Verification items for the finished model (mm, model axes). Face numbers are marked on the shaded views. A direction names the side the tool comes from. Round coordinates to 2 decimals unless told otherwise and drop trailing zeros. Loops run counter-clockwise (first coordinate to the right, second up) from the corner with the lowest first, then second, coordinate; pieces in that order, holes last.
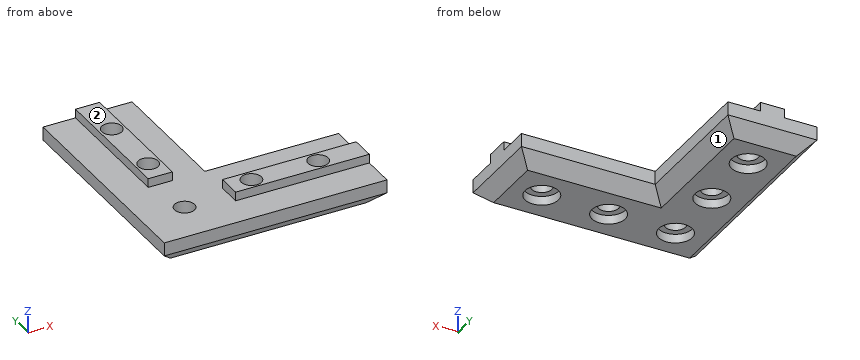
from build123d import *

# Parameters (mm, degrees)
F1_DEPTH = 6
F3_DEPTH = 2
F4_R     = 2.25
F5_DEPTH = 8.001
F6_R     = 3.75
F7_DEPTH = 2
F8_SIZE  = 3


with BuildPart() as f1:
    # F0 (on Top) → F1 (new body)
    with BuildSketch(Plane.XY):
        Polygon((0, 50), (0, 0), (50, 0), (50, 20), (20, 20), (20, 50), align=None)
    extrude(amount=F1_DEPTH)

    # F2 (on face) → F3 (join)
    with BuildSketch(Plane.XY.offset(6)):
        Polygon((12.71, 50), (7.29, 50), (7.29, 20), (10, 20), (12.71, 20), align=None)
        Polygon((50, 7.29), (50, 12.71), (20, 12.71), (20, 10), (20, 7.29), align=None)
    extrude(amount=F3_DEPTH)

    # F4 (on face) → F5 (cut, through all)
    with BuildSketch(Plane(origin=(0, 0, 0), x_dir=(1, 0, 0), z_dir=(0, 0, -1))):
        with Locations((10, -10)):
            Circle(F4_R)
        with Locations((40, -10)):
            Circle(F4_R)
        with Locations((10, -40)):
            Circle(F4_R)
        with Locations((25, -10)):
            Circle(F4_R)
        with Locations((10, -25)):
            Circle(F4_R)
    extrude(amount=-F5_DEPTH, mode=Mode.SUBTRACT)

    # F6 (on face) → F7 (cut)
    with BuildSketch(Plane(origin=(0, 0, 0), x_dir=(1, 0, 0), z_dir=(0, 0, -1))):
        with Locations((10, -10)):
            Circle(F6_R)
        with Locations((25, -10)):
            Circle(F6_R)
        with Locations((40, -10)):
            Circle(F6_R)
        with Locations((10, -25)):
            Circle(F6_R)
        with Locations((10, -40)):
            Circle(F6_R)
    extrude(amount=-F7_DEPTH, mode=Mode.SUBTRACT)

    # F8
    f8_edges = [f1.edges().sort_by_distance(p)[0] for p in [
        (25, 0, 0),
        (0, 25, 0),
        (20, 35, 0),
        (35, 20, 0),
        (50, 10, 0),
        (10, 50, 0),
    ]]
    chamfer(f8_edges, length=F8_SIZE)


solid = f1.part
1. Scan lines: L1, parallel to Y at x = 10, z = 6.8; L2, parallel to X at y = 10, z = 4.15; L3, parallel to Y at x = 25, z = 6.55. Record each from-to range of solid material in increasing order.
2. Tool access check on the marked faces 1 and 2. Record the directions out of +Z, -Z, +X, -X, +Y, -Y that give a thin tool (end or side, any length) a straight path to the whole face; none if there is none.
3. Section check A-A (z = 7). Enter the section's corners in (x, y), then the cut area to 3 significant figures.
4. Section check D-D (y = 10). Give the number of separate pieces and of enclosed holes in the cut face, then the cut area to 3 significant figures.
5. Section check B-B (y = 25). Enter the section's corners in (x, z).
6. Gauge pin test, flat ends, axial feed: P1, Ø2.5, axis at y = 42, z = 4.5, coming from the +X side; P2, Ø3, axis at x = 27, z = 2.5, coming from the +Y side; P3, Ø1, axis at x = 31.5, z = 7, coming from the -Y side. Record the tip position at first contact, or that the pin passes through.
Taken from the geometry:
1. L1: y = 20 to 22.75, 27.25 to 37.75, 42.25 to 50
1. L2: x = 0 to 7.75, 12.25 to 22.75, 27.25 to 37.75, 42.25 to 50
1. L3: y = 7.29 to 7.75, 12.25 to 12.71
2. face 1: -Z, +X, +Y
2. face 2: +Z, +X, -X, +Y, -Y
3. outline: (7.29, 20) - (12.71, 20) - (12.71, 50) - (7.29, 50) - close; (20, 7.29) - (50, 7.29) - (50, 12.71) - (20, 12.71) - close; hole circle Ø4.5 at (10, 25); hole circle Ø4.5 at (10, 40); hole circle Ø4.5 at (25, 10); hole circle Ø4.5 at (40, 10)
3. area: 262 mm2
4. separate pieces: 4
4. enclosed holes: 0
4. area: 234 mm2
5. outline: (0, 3) - (3, 0) - (6.25, 0) - (6.25, 2) - (7.75, 2) - (7.75, 8) - (7.29, 8) - (7.29, 6) - (0, 6) - close; (12.25, 2) - (13.75, 2) - (13.75, 0) - (17, 0) - (20, 3) - (20, 6) - (12.71, 6) - (12.71, 8) - (12.25, 8) - close
6. P1: stops at x = 20
6. P2: stops at y = 20
6. P3: stops at y = 7.29
